Can you work these out from the model? Positions are in its coordinate system, mm. Face numbers are marked on the shaded views. Coordinates: 2 decimals unless noted, no trailing zeros. Order: outer loops, then holes, each group sorted by start corner. A loop starts at its lowest first (then second) coordinate and runs counter-clockwise, first axis right, second up.
```python
from build123d import *


with BuildPart() as part:
    # Szkic1 → Obrót1 (revolve)
    with BuildSketch(Plane.XY, mode=Mode.PRIVATE) as obr_t1_sk:
        with BuildLine():
            Line((-17.5, 15.4), (-17.5, 0.6))
            ThreePointArc((-17.5, 0.6), (-17.324264069, 0.175735931), (-16.9, 0))
            Line((-16.9, 0), (-8.1, 0))
            ThreePointArc((-8.1, 0), (-7.675735931, 0.175735931), (-7.5, 0.6))
            Line((-7.5, 0.6), (-7.5, 15.4))
            ThreePointArc((-7.5, 15.4), (-7.675735931, 15.824264069), (-8.1, 16))
            Line((-8.1, 16), (-16.9, 16))
            ThreePointArc((-16.9, 16), (-17.324264069, 15.824264069), (-17.5, 15.4))
        make_face()
    revolve(obr_t1_sk.sketch.rotate(Axis((0, 0, 0), (0, 1, 0)), 270), axis=Axis((0, 0, 0), (0, 1, 0)))


solid = part.part
```
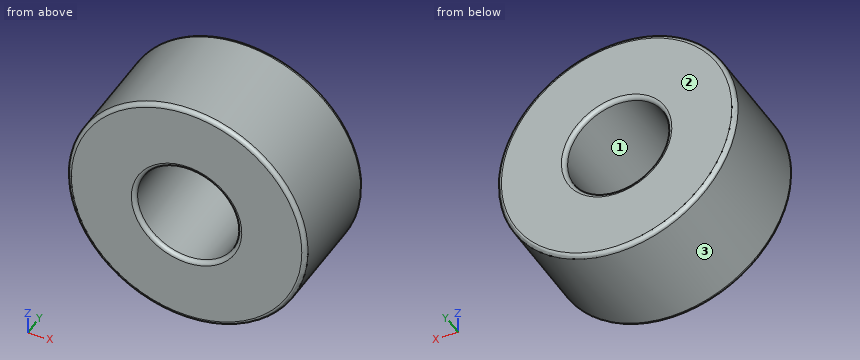
1. Thinking about a two-plate mould opening in Z: for the marked faces 1, 2 and 3, which applies, pulls with the +Z half, pulls with the -Z half, needs draft (parallel to the pull), parting line crosses it, or undercut?
Completed:
face 1: undercut
face 2: needs draft
face 3: parting line crosses it
2. Imagine slicing it at A-A on z = 0. Please give me the cut outline in (x, y), then the cut area to 3 significant figures.
Completed:
outline: (-17.5, 0.6) arc R0.6 ccw to (-16.9, 0) - (-8.1, 0) arc R0.6 ccw to (-7.5, 0.6) - (-7.5, 15.4) arc R0.6 ccw to (-8.1, 16) - (-16.9, 16) arc R0.6 ccw to (-17.5, 15.4) - close; (7.5, 0.6) arc R0.6 ccw to (8.1, 0) - (16.9, 0) arc R0.6 ccw to (17.5, 0.6) - (17.5, 15.4) arc R0.6 ccw to (16.9, 16) - (8.1, 16) arc R0.6 ccw to (7.5, 15.4) - close
area: 319 mm2
3. I'm going to push flat-ended pins straight in: pin 1 (8 mm diameter, centred on x = -1, y = 14, fed in from +Z); pin 2 (1 mm diameter, centred on y = 12.5, z = -5.5, fed in from -X); pin 3 (3 mm diameter, centred on x = -4, y = 7.5, fed in from +Z); pin 4 (6 mm diameter, centred on x = -4, y = 3, fed in from -Z). Where does each tip first touch, or does it pass through?
Completed:
pin 1: stops at z = 17.5
pin 2: stops at x = -16.77
pin 3: stops at z = 17.32
pin 4: stops at z = -17.47
4. Imagine slicing it at C-C on y = 14.75. Please give me the cut outline in (x, z), then the cut area to 3 significant figures.
Completed:
outline: circle Ø35 at (0, 0); hole circle Ø15 at (0, 0)
area: 785 mm2
5. Please list where these lines run through material, in increasing order: probe 1 along X at (y, z) = (5.5, 0); probe 2 along X at (y, z) = (13.25, 6); probe 3 along Z at (x, y) = (-5, 10.5).
Completed:
probe 1: x = -17.5 to -7.5, 7.5 to 17.5
probe 2: x = -16.44 to -4.5, 4.5 to 16.44
probe 3: z = -16.77 to -5.59, 5.59 to 16.77
6. Imagine slicing it at B-B on x = 0. Please give me the cut outline in (y, z), then the cut area to 3 significant figures.
Completed:
outline: (0, -16.9) arc R0.6 ccw to (0.6, -17.5) - (15.4, -17.5) arc R0.6 ccw to (16, -16.9) - (16, -8.1) arc R0.6 ccw to (15.4, -7.5) - (0.6, -7.5) arc R0.6 ccw to (0, -8.1) - close; (0, 8.1) arc R0.6 ccw to (0.6, 7.5) - (15.4, 7.5) arc R0.6 ccw to (16, 8.1) - (16, 16.9) arc R0.6 ccw to (15.4, 17.5) - (0.6, 17.5) arc R0.6 ccw to (0, 16.9) - close
area: 319 mm2
